Design review of the part built by this model. Coordinates are the model's own, in mm. Round coordinates to 2 decimals unless told otherwise and drop trailing zeros. Loops run counter-clockwise (first coordinate to the right, second up) from the corner with the lowest first, then second, coordinate; pieces in that order, holes last. Notation, with made-up numbers: (3.25, 62) - (12.25, 62) arc R27 cw to (12.25, 92) - close; hole circle Ø9 at (69.5, -12). An arc over 180 degrees is marked (long way). Use one line per item in the form item = value. Start each with the question number.
(1) We need section A-A, the plane y = 19.25. Write out the cut boundary in (x, z).
(2) For pin 1 (8 mm diameter, centred on y = 12.7, z = 438.15, fed in from -X), flat-tipped, find the tip position at first contact; note if it passes through.
(3) Wall thickness on probe 1 along Y at (x, z) = (24.75, 438.15); probe 2 along X at (y, z) = (11.5, 293): over which ranges is each line inside the solid? List them lowest first. Write a range as [from, to].
(4) We need section B-B, the plane z = 297.5. Write out the cut boundary in (x, y).
from build123d import *

# Parameters (mm, degrees)
SKETCH1_W           = 25.4
SKETCH1_H           = 25.4
SKETCH1_W_2         = 22.225
SKETCH1_H_2         = 22.225
BOSS_EXTRUDE1_DEPTH = 450.85
SKETCH4_R           = 2.54
CUT_EXTRUDE3_DEPTH  = 453.278722139
SKETCH5_R           = 2.54
CUT_EXTRUDE4_DEPTH  = 453.278722139


with BuildPart() as part:
    # Sketch1 → Boss-Extrude1 (new body)
    with BuildSketch(Plane.XY):
        with Locations((12.7, 12.7)):
            Rectangle(SKETCH1_W, SKETCH1_H)
        with Locations((12.7, 12.7)):
            Rectangle(SKETCH1_W_2, SKETCH1_H_2, mode=Mode.SUBTRACT)
    extrude(amount=BOSS_EXTRUDE1_DEPTH)

    # Sketch4 → Cut-Extrude3 (cut, through all)
    with BuildSketch(Plane(origin=(25.4, 0, 0), x_dir=(0, 0, -1), z_dir=(1, 0, 0))):
        with Locations((-438.15, 12.7)):
            Circle(SKETCH4_R)
        with Locations(Location((-12.7, 12.7, 0), (0, 0, 180))):
            Circle(SKETCH4_R)
    extrude(amount=-CUT_EXTRUDE3_DEPTH, mode=Mode.SUBTRACT)

    # Sketch5 → Cut-Extrude4 (cut, through all)
    with BuildSketch(Plane.XZ):
        with Locations(Location((11.1125, 438.15, 0), (0, 0, 270))):
            Circle(SKETCH5_R)
        with Locations(Location((11.1125, 12.7, 0), (0, 0, 270))):
            Circle(SKETCH5_R)
    extrude(amount=-CUT_EXTRUDE4_DEPTH, mode=Mode.SUBTRACT)


solid = part.part
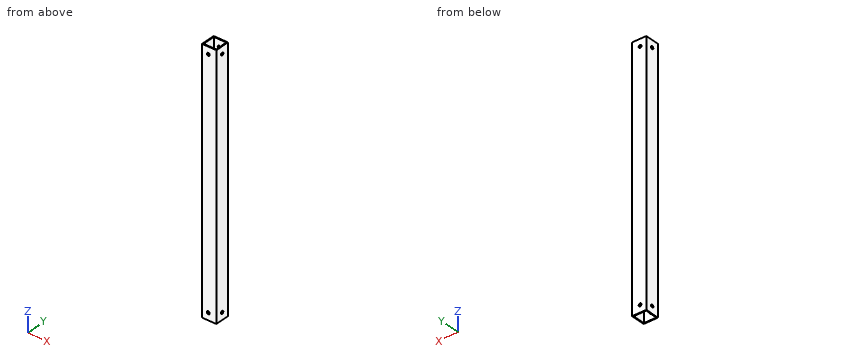
Data:
q1.outline = (0, 0) - (1.59, 0) - (1.59, 450.85) - (0, 450.85) - close; (23.81, 0) - (25.4, 0) - (25.4, 450.85) - (23.81, 450.85) - close
q2.pin_1 = 0
q3.probe_1 = [0, 10.16], [15.24, 25.4]
q3.probe_2 = [0, 1.59], [23.81, 25.4]
q4.outline = (0, 0) - (25.4, 0) - (25.4, 25.4) - (0, 25.4) - close; hole (1.59, 1.59) - (23.81, 1.59) - (23.81, 23.81) - (1.59, 23.81) - close
